from build123d import *

# Parameters (mm, degrees)
SKETCH1_W  = 64.999999997
SKETCH1_H  = 11.938
SKETCH13_W = 5.08
SKETCH13_H = 2.032


with BuildPart() as part:
    # Sketch1 → Blank (revolve)
    with BuildSketch(Plane.XY):
        with Locations((-32.499999999, 0)):
            Rectangle(SKETCH1_W, SKETCH1_H)
    revolve(axis=Axis((0, 5.969, 0), (0, -1, 0)))

    # Sketch7 → Single Side Bore (revolve, cut)
    with BuildSketch(Plane.XY, mode=Mode.PRIVATE) as single_side_bore_sk:
        Polygon((-23.749, -5.969), (-23.749, 2.159), (-51.029999997, 2.159), (-51.029999997, 5.969), (0, 5.969), (0, -5.969), align=None)
    revolve(single_side_bore_sk.sketch.rotate(Axis((0, 5.969, 0), (0, 1, 0)), 270), axis=Axis((0, 5.969, 0), (0, 1, 0)), mode=Mode.SUBTRACT)



with BuildPart() as body_2:
    # Sketch9 → KF Flange (revolve)
    with BuildSketch(Plane.XY, mode=Mode.PRIVATE) as kf_flange_sk:
        Polygon((30.355443212, -35.251), (23.749, -35.251), (23.749, -37.7148), (26.1239, -37.7148), (26.1239, -40.331), (37.465, -40.331), (37.465, -37.156), align=None)
    revolve(kf_flange_sk.sketch.rotate(Axis((0, 5.969, 0), (0, -1, 0)), 180), axis=Axis((0, 5.969, 0), (0, -1, 0)))


with BuildPart() as part_1:
    add(part.part)

    add(body_2.part)  # Revolve1 merges body 2
    # Sketch8 → Revolve1 (revolve)
    with BuildSketch(Plane.XY, mode=Mode.PRIVATE) as revolve1_sk:
        Polygon((-23.749, 2.159), (-23.749, -13.081), (-23.749, -22.4748), (-23.749, -37.7148), (-25.4, -37.7148), (-25.4, -22.4748), (-25.4, -13.081), (-25.4, 2.159), align=None)
    revolve(revolve1_sk.sketch.rotate(Axis((0, 0, 0), (0, -1, 0)), 180), axis=Axis((0, 0, 0), (0, -1, 0)))

    # Sketch13 → Cut-Revolve2 (revolve, cut)
    with BuildSketch(Plane.XY, mode=Mode.PRIVATE) as cut_revolve2_sk:
        with Locations((-59.919999997, -4.953)):
            Rectangle(SKETCH13_W, SKETCH13_H)
    revolve(cut_revolve2_sk.sketch.rotate(Axis((0, 0, 0), (0, -1, 0)), 270), axis=Axis((0, 0, 0), (0, -1, 0)), mode=Mode.SUBTRACT)

    # Sketch15 → Cut-Revolve3 (revolve, cut)
    with BuildSketch(Plane.XY):
        with BuildLine():
            Line((-64.999999997, 2.286), (-64.999999997, -0.889))
            ThreePointArc((-64.999999997, -0.889), (-63.412499997, 0.6985), (-64.999999997, 2.286))
        make_face()
    revolve(axis=Axis((0, 0, 0), (0, -1, 0)), mode=Mode.SUBTRACT)


solid = part_1.part
Model file for the job. Use its own axes, mm. A direction names the side the tool comes from. Give positions to 0.01 mm unless a question says otherwise; leave off trailing zeros. Answer as CSV lines item,"result".
1. Drill centre lines: L1, parallel to Y at x = 21, z = -17.5; L2, parallel to Z at x = 1, y = -31; L3, parallel to Z at x = 0, y = -38.65 (3 decimals). Where is each one in solid material? Low to high. Write a range as [from, to].
Responses:
L1,"y = [-40.33, -35.25], [-5.97, 2.16]"
L2,"z = [-25.38, -23.73], [23.73, 25.38]"
L3,"z = [-37.465, -26.124], [26.124, 37.465]"
2. Pin check, flat tips, straight feed: pin 1 (4 mm diameter, centred on y = 1.5, z = -19.5, fed in from -X); pin 2 (10 mm diameter, centred on x = 44, z = -44.5, fed in from -Y); pin 3 (10 mm diameter, centred on x = -12.5, y = -7.5, fed in from +Z). Stop position of each tip, or through.
Responses:
pin 1,"stops at x = -62.55"
pin 2,"stops at y = -5.97"
pin 3,"stops at z = 64.54"
3. 3-axis set-ups, long thin cutter, end or side, ignore diameter. For faces 4 (the face through (31.051, 4.091, 40.496)), 5 (the face through (7, -35.251, 25)), 6 (the face through (-17.24, -4.94, 54.73)): which of +Z, -Z, +X, -X, +Y, -Y reach the whole face in a straight line?
Responses:
face 4,"+Y"
face 5,"none"
face 6,"-Y"
4. Two-plate mould, pull along Y, no slides. Class faces 1 (the face through (-18.761, -4.939, 59.576)), 2 (the face through (51, -3.937, 27)), 3 (the face through (-12, -5.969, 25)): +Y half, -Y half, draft (parallel to the pull), parting line (faces both ways), or undercut.
Responses:
face 1,"draft"
face 2,"-Y half"
face 3,"undercut"
